The listing builds one solid part. Answer for the finished solid, in the listing's coordinates (mm). Give positions to 0.01 mm unless a question says otherwise; leave off trailing zeros. Write each loop counter-clockwise with the first axis right and the second up, starting at its lowest first coordinate (ties: lowest second). Pieces come first, ordered by that corner, then holes. Notation, with made-up numbers: (2, 52.5) -> (9, 52.5) arc R13 cw to (9, 66.5) -> close; hole circle Ø10 at (61, -18). An arc over 180 degrees is marked (long way). One line per question, with ' | ' between items.
Autodesk Inventor part; units mm, degrees
ref_plane "YZ Plane" through (0, 0, 0) normal (1, 0, 0) x (0, 1, 0)
ref_plane "XZ Plane" through (0, 0, 0) normal (0, 1, 0) x (-1, 0, 0)
ref_plane "XY Plane" through (0, 0, 0) normal (0, 0, 1) x (1, 0, 0)
sketch "Schizzo1" plane through (0, 0, 0) normal (0, 0, 1) x (1, 0, 0)
  circle A0 centre (0, 0) radius 150
  circle A1 centre (0, 0) radius 75
  circle A2 centre (-120, 0) radius 10
  circle A3 centre (-84.8528, 84.8528) radius 10
  circle A4 centre (0, 120) radius 10
  circle A5 centre (84.8528, 84.8528) radius 10
  circle A6 centre (120, 0) radius 10
  circle A7 centre (84.8528, -84.8528) radius 10
  circle A8 centre (0, -120) radius 10
  circle A9 centre (-84.8528, -84.8528) radius 10
  dimension "d0" = 150
  dimension "d1" = 300
  dimension "d2" = 20
  dimension "d5" = 360
  dimension "d9" = 120
extrude "Estrusione1" add sketch "Schizzo1" along normal mid plane 20
properties part number "05-22-2023 flangia"
Item 1: Find section D-D (z = -3). Count the separate pieces of the cut face and the enclosed holes in it, then the cut area to 3 significant figures.
Answers below:
separate pieces: 1 | enclosed holes: 9 | area: 50,500 mm²
Item 2: Flat-ended cylindrical pins translate along their axes: pin 1 (18 mm diameter, centred on x = -120, y = 0, fed in from +Z); pin 2 (6 mm diameter, centred on x = -62.5, z = -1, fed in from -Y); pin 3 (23 mm diameter, centred on x = 0, y = 120, fed in from +Z); pin 4 (1 mm diameter, centred on y = 89.5, z = -8, fed in from -X). Find the tip coordinate at first contact, or state that the pin passes through.
Answers below:
pin 1: through | pin 2: y = -137.69 | pin 3: z = 10 | pin 4: x = -120.74
Item 3: Find section B-B (y = -120). Write down the section's boundary in (x, z), then the cut area to 3 significant figures.
Answers below:
outline: (-90, -10) -> (-10, -10) -> (-10, 10) -> (-90, 10) -> close; (10, -10) -> (90, -10) -> (90, 10) -> (10, 10) -> close | area: 3,200 mm²
Item 4: Consider line 1 (Y direction, x = 0, z = 3.25); line 2 (Y direction, x = 85.5, z = -7); line 3 (Y direction, x = 81, z = 2). Determine where each line is inside the solid, lowest interval first. Write a range as [from, to].
Answers below:
line 1: [-150, -130], [-110, -75], [75, 110], [130, 150] | line 2: [-123.25, -94.83], [-74.87, 74.87], [94.83, 123.25] | line 3: [-126.25, -94.08], [-75.62, 75.62], [94.08, 126.25]
Item 5: Determine the mould class of faces 1 (the face through (-69, -31, 10)), 2 (the face through (-19.527, 148.724, 0.14)), 3 (the face through (-75.615, 81.023, 0.14)) for opening direction X: pulls with the +X half, pulls with the -X half, needs draft (parallel to the pull), parting line crosses it, or undercut.
Answers below:
face 1: needs draft | face 2: parting line crosses it | face 3: undercut
Item 6: Find section A-A (y = 0). Write down the section's boundary in (x, z), then the cut area to 3 significant figures.
Answers below:
outline: (-150, -10) -> (-130, -10) -> (-130, 10) -> (-150, 10) -> close; (-110, -10) -> (-75, -10) -> (-75, 10) -> (-110, 10) -> close; (75, -10) -> (110, -10) -> (110, 10) -> (75, 10) -> close; (130, -10) -> (150, -10) -> (150, 10) -> (130, 10) -> close | area: 2,200 mm²
